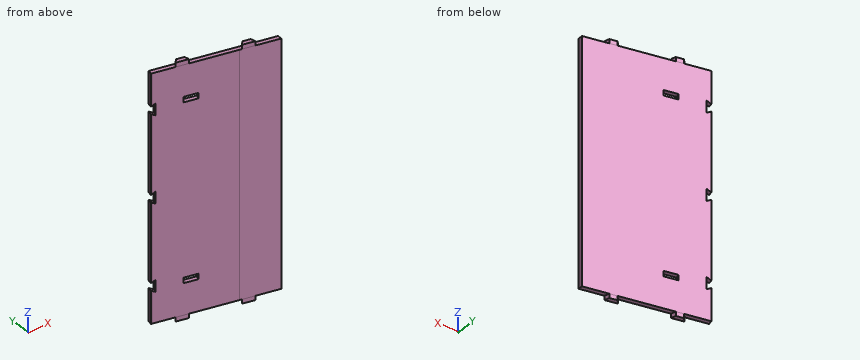
from build123d import *

# Parameters (mm, degrees)
F1_DEPTH  = 203.5
F3_DEPTH  = 3.5
F4_DEPTH  = 210.5
F6_DEPTH  = 25
F7_W      = 10
F7_H      = 4.5
F8_DEPTH  = 25
F9_DEPTH  = 0.5
F10_DEPTH = 0.5


with BuildPart() as f1:
    # F0 (on Top) → F1 (new body)
    with BuildSketch(Plane.XY):
        Polygon((18.1093649228, 1.9817664346), (80.342321908, -12.1293889498), (110.342321908, -18.9318081509), (110.342321908, -15.3429607484), (18.1093649228, 5.5706138371), (17.3353965158, 2.1572616864), align=None)
    extrude(amount=F1_DEPTH)

    # F2 (on face) → F3 (join)
    with BuildSketch(Plane.XY.offset(203.5)):
        Polygon((43.4656951855, -0.1788657578), (37.6142343556, 1.1479372257), (34.8897790053, -1.8231472639), (44.6422137217, -4.0344855696), align=None)
        Polygon((90.8374524752, -10.9202841369), (84.9859916454, -9.5934811535), (82.2615362951, -12.5645656431), (92.0139710115, -14.7759039488), align=None)
    extrude(amount=F3_DEPTH)

    # F4 (add): faces of the model
    f4_faces = [f1.faces().sort_by_distance(p)[0] for p in [
        (40.1207318834, -1.3643633477, 207),
        (87.4924891732, -12.1057817269, 207),
    ]]
    extrude(f4_faces, amount=-F4_DEPTH)

    # F5 (on face) → F6 (cut)
    with BuildSketch(Plane(origin=(2.0869058597, 9.2036632764, 0), x_dir=(-0.9752434716, 0.2211338306, 0), z_dir=(0.2211338306, 0.9752434716, 0))):
        Polygon((-16.4291887401, 170.5), (-16.4291887401, 176.5), (-19.9291887401, 178.5), (-19.9291887401, 168.5), align=None)
        Polygon((-16.4291887401, 101.75), (-16.4291887401, 104.75), (-19.9291887401, 106.75), (-19.9291887401, 101.75), (-19.9291887401, 96.75), (-16.4291887401, 98.75), align=None)
        Polygon((-16.4291887401, 27), (-16.4291887401, 33), (-19.9291887401, 35), (-19.9291887401, 25), align=None)
    extrude(amount=-F6_DEPTH, mode=Mode.SUBTRACT)

    # F7 (on face) → F8 (cut)
    with BuildSketch(Plane(origin=(1.3129374527, 5.7903111257, 0), x_dir=(0.9752434716, -0.2211338306, 0), z_dir=(-0.2211338306, -0.9752434716, 0))):
        with Locations((45.8121887401, 175.25)):
            Rectangle(F7_W, F7_H)
        with Locations((45.8121887401, 28.25)):
            Rectangle(F7_W, F7_H)
    extrude(amount=-F8_DEPTH, mode=Mode.SUBTRACT)

    # F9 (cut): faces of the model
    f9_faces = [f1.faces().sort_by_distance(p)[0] for p in [
        (41.5017422883, -1.5279684291, 175.25),
        (41.5017422883, -1.5279684291, 28.25),
    ]]
    extrude(f9_faces, amount=-F9_DEPTH, mode=Mode.SUBTRACT)

    # F10 (cut): faces of the model
    f10_faces = [f1.faces().sort_by_distance(p)[0] for p in [
        (51.2541770047, -3.7393067348, 175.25),
        (51.2541770047, -3.7393067348, 28.25),
    ]]
    extrude(f10_faces, amount=-F10_DEPTH, mode=Mode.SUBTRACT)


solid = f1.part
Geometry check sheet. Reference: the model listing, model coordinates, mm. Coordinates: 2 decimals unless noted, no trailing zeros. Write each loop counter-clockwise with the first axis right and the second up, starting at its lowest first coordinate (ties: lowest second). Pieces come first, ordered by that corner, then holes. Notation, with made-up numbers: (1, 58) -> (34, 58) arc R32 ccw to (34, 88) -> close; hole circle Ø6 at (20.5, 60). An arc over 180 degrees is marked (long way). One line per question, with ' | ' between items.
1. Thickness scan on probe 1 along Z at (x, y) = (79, -8.5); probe 2 along Y at (x, z) = (91, 110.5); probe 3 along Y at (x, z) = (72, 54). Record the ranges inside material, lowest first. Write a range as from..to.
Answers:
probe 1: z = 0..203.5 | probe 2: y = -14.55..-10.96 | probe 3: y = -10.24..-6.65
2. Cross-section at A-A on x = 47. Record the cut outline in (y, z).
Answers:
outline: (-4.57, 0) -> (-0.98, 0) -> (-0.98, 26) -> (-4.57, 26) -> close; (-4.57, 30.5) -> (-0.98, 30.5) -> (-0.98, 173) -> (-4.57, 173) -> close; (-4.57, 177.5) -> (-0.98, 177.5) -> (-0.98, 203.5) -> (-4.57, 203.5) -> close
3. Cross-section at C-C on x = 60.5. Record the cut outline in (y, z), and give its area (3 significant figures).
Answers:
outline: (-7.63, 0) -> (-4.04, 0) -> (-4.04, 203.5) -> (-7.63, 203.5) -> close | area: 730 mm²
4. Cross-section at B-B on z = 158.5. Record the cut outline in (x, y).
Answers:
outline: (17.34, 2.16) -> (110.34, -18.93) -> (110.34, -15.34) -> (18.11, 5.57) -> close
5. Depth check by flat-ended pin: pin 1 Ø4 at (x, y) = (99, -14.5) entering from +Z; pin 2 Ø3.5 at (x, y) = (28, 1.5) entering from -Z; pin 3 Ø3 at (x, z) = (98, 115) entering from -Y; pin 4 Ø6.5 at (x, y) = (44.5, -2) entering from +Z. Enter the tip coordinate at first touch or a pass-through.
Answers:
pin 1: stops at z = 203.5 | pin 2: stops at z = 0 | pin 3: stops at y = -16.47 | pin 4: stops at z = 207
